from build123d import *

# Parameters (mm, degrees)
SKETCH_2_W                   = 35
SKETCH_2_H                   = 40
EXTRUDE_1_DEPTH              = 8
SKETCH_3_R                   = 2
CUT_EXTRUDE_2_DEPTH          = 10
SKETCH_4_W                   = 15
SKETCH_4_H                   = 40
EXTRUDE_2_DEPTH              = 24
SKETCH_5_R                   = 6.2
CUT_EXTRUDE_3_DEPTH          = 46.265881191
SKETCH_6_R                   = 10
CUT_EXTRUDE_4_DEPTH          = 3
FILLET_2_R                   = 3
FILLET_3_R                   = 10
HOLE_WIZARD_M4_1_D           = 4.3
HOLE_WIZARD_M4_1_DEPTH       = 8
HOLE_WIZARD_M4_1_CSINK_D     = 8.96
HOLE_WIZARD_M4_1_CSINK_ANGLE = 90
SKETCH_9_R                   = 10
EXTRUDE_3_DEPTH              = 3
SKETCH_10_R                  = 4.25
CUT_EXTRUDE_5_DEPTH          = 3
CUT_EXTRUDE_6_DEPTH          = 5
SKETCH_14_R                  = 6.2
SKETCH_14_R_2                = 4.25
EXTRUDE_4_DEPTH              = 12
SKETCH_15_R                  = 2
CUT_EXTRUDE_8_DEPTH          = 22


with BuildPart() as part:
    # 草图2 → 凸台-拉伸1 (new body)
    with BuildSketch(Plane(origin=(0, 0, 0), x_dir=(1, 0, 0), z_dir=(0, 1, 0))):
        Rectangle(SKETCH_2_W, SKETCH_2_H)
    extrude(amount=EXTRUDE_1_DEPTH)

    # 草图3 → 切除-拉伸2 (cut)
    with BuildSketch(Plane(origin=(0, 8, 0), x_dir=(1, 0, 0), z_dir=(0, 1, 0))):
        with Locations(Location((12.5, 15, 0), (0, 0, 270))):
            Circle(SKETCH_3_R)
        with Locations(Location((-12.5, 15, 0), (0, 0, 270))):
            Circle(SKETCH_3_R)
        with Locations(Location((-12.5, -15, 0), (0, 0, 270))):
            Circle(SKETCH_3_R)
        with Locations(Location((12.5, -15, 0), (0, 0, 270))):
            Circle(SKETCH_3_R)
    extrude(amount=-CUT_EXTRUDE_2_DEPTH, mode=Mode.SUBTRACT)

    # 草图4 → 凸台-拉伸2 (add)
    with BuildSketch(Plane(origin=(0, 8, 0), x_dir=(1, 0, 0), z_dir=(0, 1, 0))):
        Rectangle(SKETCH_4_W, SKETCH_4_H)
    extrude(amount=EXTRUDE_2_DEPTH)

    # 草图5 → 切除-拉伸3 (cut, through all)
    with BuildSketch(Plane(origin=(7.5, 0, 0), x_dir=(0, 0, -1), z_dir=(1, 0, 0))):
        with Locations((0, 18)):
            Circle(SKETCH_5_R)
    extrude(amount=-CUT_EXTRUDE_3_DEPTH, mode=Mode.SUBTRACT)

    # 草图6 → 切除-拉伸4 (cut)
    with BuildSketch(Plane(origin=(7.5, 0, 0), x_dir=(0, 0, -1), z_dir=(1, 0, 0))):
        with Locations((0, 18)):
            Circle(SKETCH_6_R)
    extrude(amount=-CUT_EXTRUDE_4_DEPTH, mode=Mode.SUBTRACT)

    # 圆角2
    fillet_2_edges = [part.edges().sort_by_distance(p)[0] for p in [
        (17.5, 4, -20),
        (-17.5, 4, -20),
        (-17.5, 4, 20),
        (17.5, 4, 20),
    ]]
    fillet(fillet_2_edges, radius=FILLET_2_R)

    # 圆角3
    fillet_3_edges = [part.edges().sort_by_distance(p)[0] for p in [
        (0, 32, 20),
        (0, 32, -20),
    ]]
    fillet(fillet_3_edges, radius=FILLET_3_R)

    # M4 六角凹锥坑螺钉的锥形沉头孔1
    with Locations(Plane(origin=(0, 8, 0), x_dir=(1, 0, 0), z_dir=(0, 1, 0))):
        with Locations((12.5, -15), (12.5, 15), (-12.5, 15), (-12.5, -15)):
            CounterSinkHole(HOLE_WIZARD_M4_1_D / 2, HOLE_WIZARD_M4_1_CSINK_D / 2, depth=HOLE_WIZARD_M4_1_DEPTH, counter_sink_angle=HOLE_WIZARD_M4_1_CSINK_ANGLE)

    # 草图9 → 凸台-拉伸3 (add)
    with BuildSketch(Plane(origin=(7.5, 0, 0), x_dir=(0, 0, -1), z_dir=(1, 0, 0))):
        with Locations((0, 18)):
            Circle(SKETCH_9_R)
    extrude(amount=-EXTRUDE_3_DEPTH)

    # 草图10 → 切除-拉伸5 (cut)
    with BuildSketch(Plane.ZY.offset(-4.5)):
        with Locations((0, 18)):
            Circle(SKETCH_10_R)
    extrude(amount=-CUT_EXTRUDE_5_DEPTH, mode=Mode.SUBTRACT)

    # 草图12 → 切除-拉伸6 (cut, symmetric)
    with BuildSketch(Plane.ZY.offset(12.5)):
        with BuildLine():
            Line((-10, 8), (10, 8))
            ThreePointArc((10, 8), (0, 4.045383588), (-10, 8))
        make_face()
    cut_extrude_6 = extrude(amount=CUT_EXTRUDE_6_DEPTH, both=True, mode=Mode.SUBTRACT)

    # 镜向1: 切除-拉伸6 across plane
    add(cut_extrude_6.mirror(Plane.ZY), mode=Mode.SUBTRACT)

    # 草图14 → 凸台-拉伸4 (add)
    with BuildSketch(Plane.ZY.offset(-4.5)):
        with Locations((0, 18)):
            Circle(SKETCH_14_R)
        with Locations((0, 18)):
            Circle(SKETCH_14_R_2, mode=Mode.SUBTRACT)
    extrude(amount=EXTRUDE_4_DEPTH)

    # 草图15 → 切除-拉伸8 (cut)
    with BuildSketch(Plane.ZY.offset(7.5)):
        with Locations((14.883032336, 20.9575309)):
            Circle(SKETCH_15_R)
    extrude(amount=-CUT_EXTRUDE_8_DEPTH, mode=Mode.SUBTRACT)


solid = part.part
Read the model definition and answer for the solid it produces. Units are mm, in the model's axes. A direction names the side the tool comes from. Coordinates: 2 decimals unless noted, no trailing zeros. Order: outer loops, then holes, each group sorted by start corner. A loop starts at its lowest first (then second) coordinate and runs counter-clockwise, first axis right, second up. Notation, with made-up numbers: (31, -1.5) - (68, -1.5) arc R27 ccw to (68, 14.5) - close; hole circle Ø5 at (-1.5, 57). An arc over 180 degrees is marked (long way). Use one line per item in the form item = value.
(1) Straight lines are drawn through the part: L1, parallel to X at y = 4, z = -15; L2, parallel to Y at x = 1, z = 0; L3, parallel to Z at x = 9.5, y = 7. For each, find the intervals that lie inside material, in ascending order.
Computed values:
L1 = -17.5 to -14.65, -10.35 to 10.35, 14.65 to 17.5
L2 = 0 to 13.75, 22.25 to 32
L3 = -20 to -16.76, -13.24 to -8.81, 8.81 to 13.24, 16.76 to 20
(2) Section D-D, the plane y = 2 is taken. Give the vertices of the cut face in (x, z), then the cut area to 3 significant figures.
Computed values:
outline = (-17.5, -17) arc R3 ccw to (-14.5, -20) - (14.5, -20) arc R3 ccw to (17.5, -17) - (17.5, 17) arc R3 ccw to (14.5, 20) - (-14.5, 20) arc R3 ccw to (-17.5, 17) - close; hole circle Ø4.3 at (-12.5, -15); hole circle Ø4.3 at (-12.5, 15); hole circle Ø4.3 at (12.5, -15); hole circle Ø4.3 at (12.5, 15)
area = 1,330 mm²
(3) Given pin 1 Ø11 at (x, z) = (-11, 15.5) entering from +Y; pin 2 Ø11 at (x, z) = (10, -15) entering from +Y; pin 3 Ø6.5 at (y, z) = (20.96, 14.88) entering from +X; pin 4 Ø6 at (y, z) = (7, 2.5) entering from +X, each flat-ended and moving along its own axis, determine where each tip first touches the part or whether it passes through.
Computed values:
pin_1 = 31.92
pin_2 = 32
pin_3 = 7.5
pin_4 = 17.5
(4) Section A-A, the plane x = -12.5 is taken. Give the vertices of the cut face in (y, z), then the cut area to 3 significant figures.
Computed values:
outline = (0, -20) - (8, -20) - (8, -19.48) - (5.67, -17.15) - (0, -17.15) - close; (0, -12.85) - (5.67, -12.85) - (8, -10.52) - (8, -10) arc R14.62 cw to (8, 10) - (8, 10.52) - (5.67, 12.85) - (0, 12.85) - close; (0, 17.15) - (5.67, 17.15) - (8, 19.48) - (8, 20) - (0, 20) - close
area = 186 mm²
(5) Which of the six approach directions +Z, -Z, +X, -X, +Y, -Y give full straight-line access (tool end or side, diameter ignored) to faces 4 (the face through (-11.459, 8, 10.486)), 5 (the face through (7.986, 8, -13.959)), 6 (the face through (12.57, 4.046, 0.154))?
Computed values:
face_4 = +Z, -Z, -X, +Y
face_5 = +Z, -Z, +X, +Y
face_6 = +X, +Y
(6) Section C-C, the plane z = 7 is taken. Give the vertices of the cut face in (x, y), then the cut area to 3 significant figures.
Computed values:
outline = (-17.5, 0) - (17.5, 0) - (17.5, 5.83) - (7.5, 5.83) - (7.5, 32) - (-7.5, 32) - (-7.5, 5.83) - (-17.5, 5.83) - close
area = 597 mm²
(7) For a pull along Z with two mould halves and no side action, classify faces 1 (the face through (-11.459, 8, -19.514)), 2 (the face through (-10.832, 5.783, -16.53)), 3 (the face through (0, 8, -20)) as pulls with the +Z half, pulls with the -Z half, needs draft (parallel to the pull), parting line crosses it, or undercut.
Computed values:
face_1 = needs draft
face_2 = undercut
face_3 = pulls with the -Z half
(8) Section B-B, the plane y = 18 is taken. Give the vertices of the cut face in (x, z), then the cut area to 4 significant figures.
Computed values:
outline = (-7.5, -20) - (7.5, -20) - (7.5, -4.25) - (-7.5, -4.25) - close; (-7.5, 4.25) - (7.5, 4.25) - (7.5, 20) - (-7.5, 20) - close
area = 472.5 mm²
